```python
from build123d import *

# Parameters (mm, degrees)
SKETCH1_R           = 50.8
SKETCH1_R_2         = 3.81
SKETCH1_R_3         = 12.7
SKETCH1_W           = 3.302
SKETCH1_H           = 19.177
BOSS_EXTRUDE1_DEPTH = 3.175


with BuildPart() as part:
    # Sketch1 → Boss-Extrude1 (new body)
    with BuildSketch(Plane(origin=(0, 0, 0), x_dir=(1, 0, 0), z_dir=(0, 1, 0))):
        Circle(SKETCH1_R)
        with Locations((-25.4, 25.4)):
            Circle(SKETCH1_R_2, mode=Mode.SUBTRACT)
        with Locations((-25.4, -25.4)):
            Circle(SKETCH1_R_2, mode=Mode.SUBTRACT)
        with Locations((25.4, -25.4)):
            Circle(SKETCH1_R_2, mode=Mode.SUBTRACT)
        with Locations((25.4, 25.4)):
            Circle(SKETCH1_R_2, mode=Mode.SUBTRACT)
        Circle(SKETCH1_R_3, mode=Mode.SUBTRACT)
        with Locations((19.431, 0)):
            Rectangle(SKETCH1_W, SKETCH1_H, mode=Mode.SUBTRACT)
        with Locations((-19.431, 0)):
            Rectangle(SKETCH1_W, SKETCH1_H, mode=Mode.SUBTRACT)
    extrude(amount=BOSS_EXTRUDE1_DEPTH)


solid = part.part
```
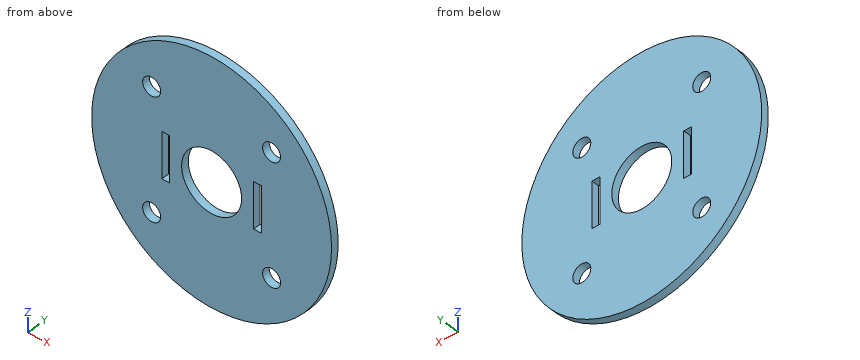
Here's how the part is built. I have some questions about the finished solid (model axes, mm). Give positions to 0.01 mm unless a question says otherwise; leave off trailing zeros. Order: outer loops, then holes, each group sorted by start corner. A loop starts at its lowest first (then second) coordinate and runs counter-clockwise, first axis right, second up. Notation, with made-up numbers: (13.25, 31) - (53.25, 31) arc R20 cw to (53.25, 40) - close; hole circle Ø4 at (89.25, 88). An arc over 180 degrees is marked (long way). Answer as a JSON object with one key per item and string values. Group by question number.
Item 1: For P1, Ø1.6, axis at x = 20, y = 1, coming from the -Z side; P2, Ø1.6, axis at y = 1, z = -4.5, coming from the -X side; P3, Ø6, axis at x = -25.4, z = 25.4, coming from the +Y side; P4, Ø1.6, axis at x = -19.5, y = 1, coming from the -Z side, each with a flat end and sliding along its axis, tell me the tip position at first contact or that it passes through.
Item 2: If we section it at C-C on x = 24: Please give me the cut outline in (y, z) (3 decimals).
Item 3: If we section it at D-D on z = 25.4: Please give me the cut outline in (x, y) (3 decimals).
Item 4: If we section it at B-B on y = 1.7: Please give me the cut outline in (x, z), and give its area (3 significant figures).
Item 5: If we section it at A-A on z = 0: Please give me the cut outline in (x, y) (3 decimals), and give its area (3 significant figures).
Item 6: Please list where these lines run through material, in increasing order: probe 1 along X at (y, z) = (2.1, 0); probe 2 along X at (y, z) = (2.3, -25.4); probe 3 along X at (y, z) = (0.95, 27.5).
Result set:
{
 "1": {"P1": "z = -47.03", "P2": "x = -50.67", "P3": "through", "P4": "z = -47.23"},
 "2": {"outline": "(0, -44.773) - (3.175, -44.773) - (3.175, -28.943) - (0, -28.943) - close; (0, -21.857) - (3.175, -21.857) - (3.175, 21.857) - (0, 21.857) - close; (0, 28.943) - (3.175, 28.943) - (3.175, 44.773) - (0, 44.773) - close"},
 "3": {"outline": "(-43.994, 0) - (-29.21, 0) - (-29.21, 3.175) - (-43.994, 3.175) - close; (-21.59, 0) - (21.59, 0) - (21.59, 3.175) - (-21.59, 3.175) - close; (29.21, 0) - (43.994, 0) - (43.994, 3.175) - (29.21, 3.175) - close"},
 "4": {"outline": "circle Ø101.6 at (0, 0); hole circle Ø7.62 at (-25.4, -25.4); hole circle Ø7.62 at (-25.4, 25.4); hole (-21.08, -9.59) - (-17.78, -9.59) - (-17.78, 9.59) - (-21.08, 9.59) - close; hole circle Ø25.4 at (0, 0); hole (17.78, -9.59) - (21.08, -9.59) - (21.08, 9.59) - (17.78, 9.59) - close; hole circle Ø7.62 at (25.4, -25.4); hole circle Ø7.62 at (25.4, 25.4)", "area": "7,290 mm²"},
 "5": {"outline": "(-50.8, 0) - (-21.082, 0) - (-21.082, 3.175) - (-50.8, 3.175) - close; (-17.78, 0) - (-12.7, 0) - (-12.7, 3.175) - (-17.78, 3.175) - close; (12.7, 0) - (17.78, 0) - (17.78, 3.175) - (12.7, 3.175) - close; (21.082, 0) - (50.8, 0) - (50.8, 3.175) - (21.082, 3.175) - close", "area": "221 mm²"},
 "6": {"probe 1": "-50.8 to -21.08, -17.78 to -12.7, 12.7 to 17.78, 21.08 to 50.8", "probe 2": "-43.99 to -29.21, -21.59 to 21.59, 29.21 to 43.99", "probe 3": "-42.71 to -28.58, -22.22 to 22.22, 28.58 to 42.71"}
}
